```python
from build123d import *

# Parameters (mm, degrees)
F_0000_CYLINDER_SKETCH_R    = 2.5
F_0000_CYLINDER_DEPTH       = 1.5
F_0001_FILLET_R             = 0.375
F_0002_EXTRUDE_DEPTH        = 0.835
F_0002_EXTRUDE_ROTATE_ANGLE = 120
F_0005_CYLINDER_SKETCH_R    = 1
F_0005_CYLINDER_DEPTH       = 9.7
F_0006_CONE_ROTATE_ANGLE    = 90


with BuildPart() as part:
    # 0000_cylinder_Sketch → 0000_cylinder (new body)
    with BuildSketch(Plane.XY):
        Circle(F_0000_CYLINDER_SKETCH_R)
    extrude(amount=F_0000_CYLINDER_DEPTH)

    # 0001_fillet
    f_0001_fillet_edges = [part.edges().sort_by_distance(p)[0] for p in [
        (-2.5, 0, 1.5),
    ]]
    fillet(f_0001_fillet_edges, radius=F_0001_FILLET_R)


with BuildPart() as body_2:
    # 0002_extrude_Sketch → 0002_extrude (new body)
    with BuildSketch(Plane.XY):
        Polygon((0, 0), (0.866025404, 0), (1.299038106, 0.75), (0.866025404, 1.5), (0, 1.5), (-0.433012702, 0.75), align=None)
    extrude(amount=F_0002_EXTRUDE_DEPTH)


with BuildPart() as body_2_1:
    # 0002_extrude_Rotate: read off the stored shape, not the designer's step
    # 0002_extrude_Rotate: moved
    add(body_2.part.rotate(Axis((0, 0, 0), (0, 0, 1)), F_0002_EXTRUDE_ROTATE_ANGLE))


with BuildPart() as body_2_2:
    # 0002_extrude_Translate: moved
    add(body_2_1.part.moved(Location((0.866025404, 0, 0.675))))


with BuildPart() as part_1:
    add(part.part)

    # 0004_sub: cut body 2
    add(body_2_2.part, mode=Mode.SUBTRACT)


with BuildPart() as body_2_2_1:
    # 0005_cylinder_Sketch → 0005_cylinder (new body)
    with BuildSketch(Plane.XY):
        Circle(F_0005_CYLINDER_SKETCH_R)
    extrude(amount=F_0005_CYLINDER_DEPTH)


with BuildPart() as body_2_2_2:
    # 0005_cylinder_Translate: moved
    add(body_2_2_1.part.moved(Location((0, 0, -9.7))))


with BuildPart() as body_3:
    # 0006_cone_Sketch → 0006_cone (revolve)
    with BuildSketch(Plane.XY, mode=Mode.PRIVATE) as f_0006_cone_sk:
        Polygon((0, 0), (1, 0), (0.7, 0.3), (0, 0.3), align=None)
    revolve(f_0006_cone_sk.sketch.rotate(Axis((0, -100, 0), (0, 1, 0)), 90), axis=Axis((0, -100, 0), (0, 1, 0)))


with BuildPart() as body_3_1:
    # 0006_cone_Rotate: moved
    add(body_3.part.rotate(Axis((0, 0, 0), (1, 0, 0)), F_0006_CONE_ROTATE_ANGLE))


with BuildPart() as body_3_2:
    # 0006_cone_Translate: moved
    add(body_3_1.part.moved(Location((0, 0, -10))))


with BuildPart() as body_2_2_3:
    add(body_2_2_2.part)

    # 0008_add: union body 3
    add(body_3_2.part)


with BuildPart() as part_2:
    add(part_1.part)

    # 0009_add: union body 2 2
    add(body_2_2_3.part)


solid = part_2.part
```
Input: part model. Units: mm. Frame: model coordinates. A direction names the side the tool comes from. Coordinates: 2 decimals unless noted, no trailing zeros. Loops run counter-clockwise (first coordinate to the right, second up) from the corner with the lowest first, then second, coordinate; pieces in that order, holes last. Notation, with made-up numbers: (63.25, -37.75) - (68.25, -37.75) arc R19 ccw to (68.25, -9.75) - close; hole circle Ø10 at (-4, 77.5). An arc over 180 degrees is marked (long way). Answer in a Markdown table with one row per item.
(1) Mould query, pull axis Y, two halves, no side actions, for faces 3 (the face through (0, -1, -5)), 4 (the face through (0, 0, 0.675)), 5 (the face through (0, -0.75, 1)), 6 (the face through (1, -1, 0)). Classes: pulls with the +Y half, pulls with the -Y half, needs draft (parallel to the pull), parting line crosses it, or undercut.
Model answer:
| item | result |
|---|---|
| face 3 | parting line crosses it |
| face 4 | undercut |
| face 5 | undercut |
| face 6 | needs draft |
(2) Set-up query: faces 1 (the face through (0, 0, -10)), 2 (the face through (0, 0.75, 1)). Return all of +Z, -Z, +X, -X, +Y, -Y with unobstructed straight access to the full face (end or side cutting, diameter ignored); none if empty.
Model answer:
| item | result |
|---|---|
| face 1 | -Z, +X, -X, +Y, -Y |
| face 2 | +Z |
(3) Pin query (flat end, axial travel): P1, Ø1, axis at x = -1, z = -7, coming from the -Y side. Return the tip coordinate at first contact, or that it passes through.
Model answer:
| item | result |
|---|---|
| P1 | stops at y = -0.87 |
(4) Cut plane A-A on x = 0. Output: boundary loops of the cut face in (y, z) (3 decimals), plus the area to 3 significant figures.
Model answer:
| item | result |
|---|---|
| outline | (-2.5, 0) - (-1, 0) - (-1, -9.7) - (-0.7, -9.7) - (-1, -10) - (1, -10) - (0.7, -9.7) - (1, -9.7) - (1, 0) - (2.5, 0) - (2.5, 1.125) arc R0.375 ccw to (2.125, 1.5) - (0.75, 1.5) - (0.75, 0.675) - (-0.75, 0.675) - (-0.75, 1.5) - (-2.125, 1.5) arc R0.375 ccw to (-2.5, 1.125) - close |
| area | 26.1 mm² |
(5) Cut plane B-B on z = -0.75. Output: boundary loops of the cut face in (x, y).
Model answer:
| item | result |
|---|---|
| outline | circle Ø2 at (0, 0) |
(6) Material intervals for L1, parallel to Z at x = -2, y = -0.7; L2, parallel to X at y = -0.5, z = -5.5, sorted ascending. Write a range as from..to.
Model answer:
| item | result |
|---|---|
| L1 | z = 0..1.5 |
| L2 | x = -0.87..0.87 |
